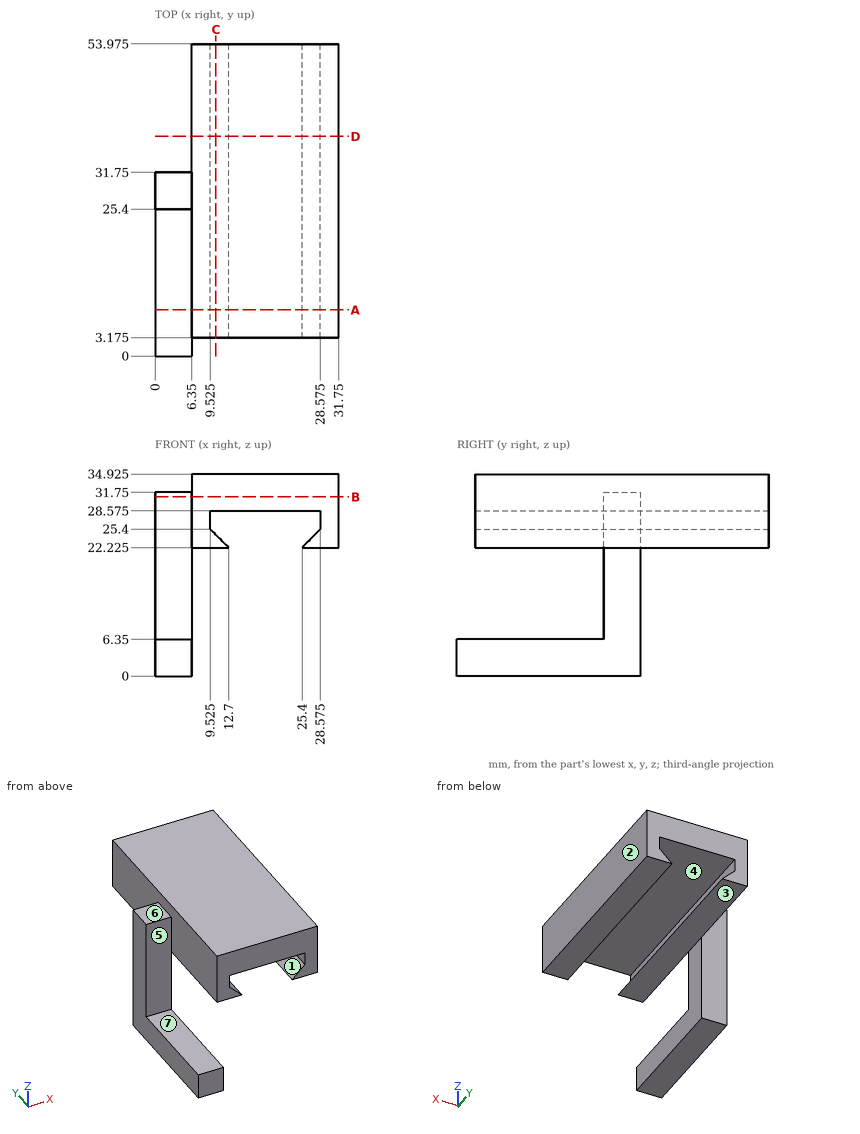
Source: three-view drawing plus pictorial views. Frame: mm from the lowest corner of the part. A direction names the side the tool comes from. Give positions to 0.01 mm unless a question says otherwise; leave off trailing zeros. Loops run counter-clockwise (first coordinate to the right, second up) from the corner with the lowest first, then second, coordinate; pieces in that order, holes last. Notation, with made-up numbers: (43.25, 25.25) -> (82.25, 25.25) arc R9 ccw to (82.25, 40.25) -> close; hole circle Ø3 at (-12, 86). An arc over 180 degrees is marked (long way). Use a Markdown table: item, result. Add a question column.
(1) Pull-direction query (X, two-part tool) for the marked faces 1, 2 and 3; classes: +X half, -X half, draft (parallel to the pull), parting line (faces both ways), or undercut.
(2) Section query A-A (y = 8). Output: boundary loops of the cut face in (x, z) (3 decimals).
(3) Section query B-B (z = 31). Output: boundary loops of the cut face in (x, y) (3 decimals).
(4) First-contact query: pin 1 Ø1 at (y, z) = (35.5, 30.5) entering from -X; pin 2 Ø18 at (y, z) = (17.5, 9) entering from +X; pin 3 Ø7 at (x, y) = (9.5, 35.5) entering from -Z (3 decimals); pin 4 Ø3 at (x, y) = (4, 48) entering from +Z. Flat tips, straight axial feed; report the tip coordinate or a pass-through.
(5) Ray query, line 1 (X direction, y = 8, z = 31.5); line 2 (Z direction, x = 7, y = 27.5) (3 decimals); line 3 (Y direction, x = 29, z = 31) (3 decimals). Return the intervals inside material, ascending.
(6) Section query C-C (x = 10.5). Output: boundary loops of the cut face in (y, z) (3 decimals).
(7) Access query for the marked faces 4, 5, 6 and 7. Directions: +Z, -Z, +X, -X, +Y, -Y. A direction counts if a zero-diameter tool reaches every point of the face in a straight line with its end or side. Return the directions, or none.
(8) Section query D-D (y = 38). Output: boundary loops of the cut face in (x, z) (3 decimals), then the cut area to 3 significant figures.
Checked values:
| question | item | result |
|---|---|---|
| 1 | face 1 | undercut |
| 1 | face 2 | +X half |
| 1 | face 3 | draft |
| 2 | outline | (0, 0) -> (6.35, 0) -> (6.35, 6.35) -> (0, 6.35) -> close; (6.35, 22.225) -> (12.7, 22.225) -> (9.525, 25.4) -> (9.525, 28.575) -> (28.575, 28.575) -> (28.575, 25.4) -> (25.4, 22.225) -> (31.75, 22.225) -> (31.75, 34.925) -> (6.35, 34.925) -> close |
| 3 | outline | (0, 25.4) -> (6.35, 25.4) -> (6.35, 3.175) -> (31.75, 3.175) -> (31.75, 53.975) -> (6.35, 53.975) -> (6.35, 31.75) -> (0, 31.75) -> close |
| 4 | pin 1 | x = 6.35 |
| 4 | pin 2 | x = 6.35 |
| 4 | pin 3 | z = 22.225 |
| 4 | pin 4 | through |
| 5 | line 1 | 6.35 to 31.75 |
| 5 | line 2 | 22.225 to 34.925 |
| 5 | line 3 | 3.175 to 53.975 |
| 6 | outline | (3.175, 22.225) -> (53.975, 22.225) -> (53.975, 24.425) -> (3.175, 24.425) -> close; (3.175, 28.575) -> (53.975, 28.575) -> (53.975, 34.925) -> (3.175, 34.925) -> close |
| 7 | face 4 | +Y, -Y |
| 7 | face 5 | +Z, -X, -Y |
| 7 | face 6 | +Z, -X, +Y, -Y |
| 7 | face 7 | +Z, +X, -X, -Y |
| 8 | outline | (6.35, 22.225) -> (12.7, 22.225) -> (9.525, 25.4) -> (9.525, 28.575) -> (28.575, 28.575) -> (28.575, 25.4) -> (25.4, 22.225) -> (31.75, 22.225) -> (31.75, 34.925) -> (6.35, 34.925) -> close |
| 8 | area | 212 mm^2 |
